Geometry: see drawing. Coordinates: mm, zero at the bounding-box minimum. A direction names the side the tool comes from. Give positions to 0.01 mm unless a question says otherwise; leave off trailing zeros. Answer as a JSON object with one key per item and string values. Group by question number.
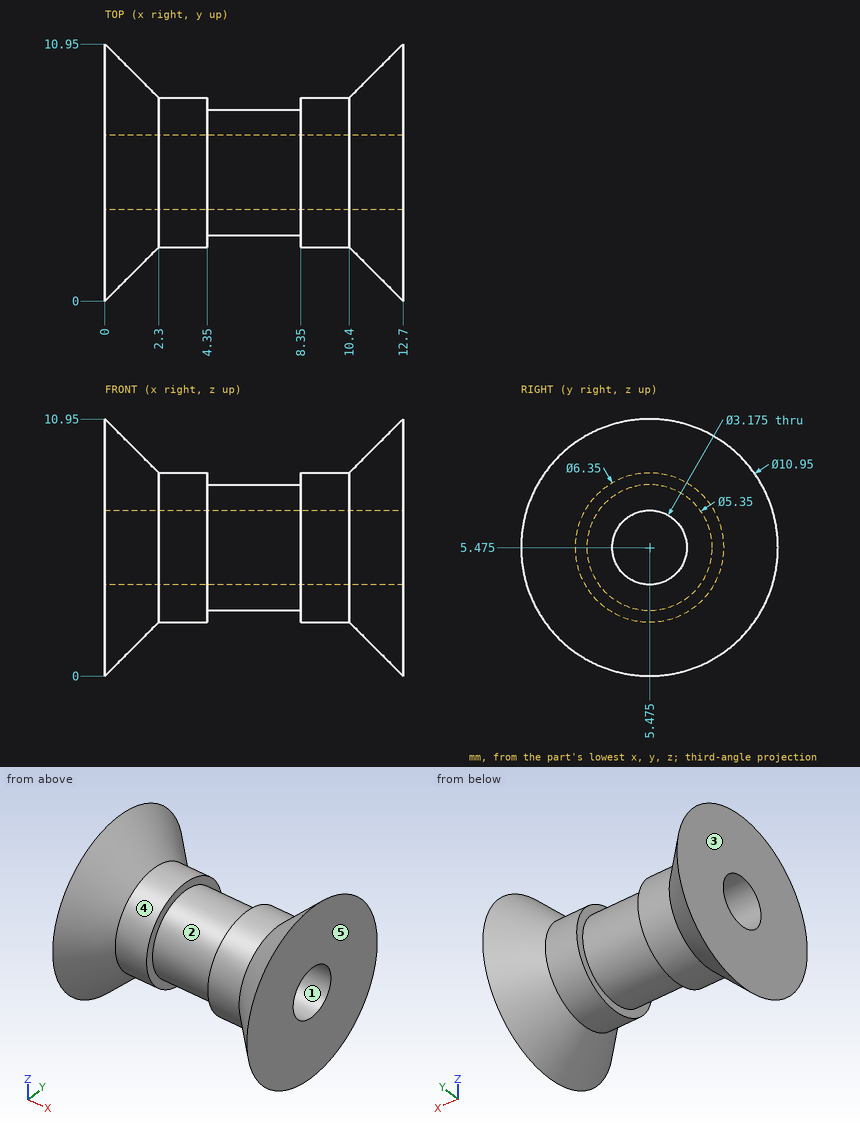
1. Line query: line 1 (Y direction, x = 7.25, z = 5.5); line 2 (X direction, y = 2.25, z = 7); line 3 (X direction, y = 4.75, z = 8.5). Output: solid intervals per line, ascending.
2. Contact query for flat-ended pins moving along their axis: pin 1 Ø2 at (x, y) = (10.5, 5) entering from +Z; pin 2 Ø1.5 at (x, y) = (5.5, 9.5) entering from -Z; pin 3 Ø2 at (x, z) = (5, 8.5) entering from -Y; pin 4 Ø3.5 at (y, z) = (5.475, 5.475) entering from -X. Output: stop coordinate, or through.
3. Reachability of the marked faces 1 and 2 from +Z, -Z, +X, -X, +Y, -Y: full face, straight path, thin tool, end or side. Return the list, or none.
4. Mould query, pull axis X, two halves, no side actions, for the marked faces 3, 4 and 5. Classes: pulls with the +X half, pulls with the -X half, needs draft (parallel to the pull), parting line crosses it, or undercut.
Working result:
{
 "1": {"line 1": "y = 2.8 to 3.89, 7.06 to 8.15", "line 2": "x = 0 to 1.91, 10.79 to 12.7", "line 3": "x = 0 to 4.35, 8.35 to 12.7"},
 "2": {"pin 1": "stops at z = 9.73", "pin 2": "passes through", "pin 3": "stops at y = 3.25", "pin 4": "stops at x = 0"},
 "3": {"face 1": "+X, -X", "face 2": "none"},
 "4": {"face 3": "pulls with the -X half", "face 4": "undercut", "face 5": "pulls with the +X half"}
}
